```python
from build123d import *

# Parameters (mm, degrees)
BOSS_EXTRUDE1_DEPTH = 2.54
SKETCH2_R           = 3.048
SKETCH2_R_2         = 1.8669
BOSS_EXTRUDE2_DEPTH = 1.1176
FILLET1_R           = 1.143
SKETCH3_R           = 1.8669
SKETCH3_R_2         = 1.42875
BOSS_EXTRUDE3_DEPTH = 1.016
SKETCH4_R           = 1.42875
CUT_EXTRUDE1_DEPTH  = 6.474765596


with BuildPart() as part:
    # Sketch1 → Boss-Extrude1 (new body)
    with BuildSketch(Plane(origin=(0, 0, 0), x_dir=(1, 0, 0), z_dir=(0, 1, 0))):
        Polygon((3.666174209, 0), (1.833087105, 3.175), (-1.833087105, 3.175), (-3.666174209, 0), (-1.833087105, -3.175), (1.833087105, -3.175), align=None)
    extrude(amount=BOSS_EXTRUDE1_DEPTH)

    # Sketch2 → Boss-Extrude2 (add)
    with BuildSketch(Plane(origin=(0, 2.54, 0), x_dir=(1, 0, 0), z_dir=(0, 1, 0))):
        with Locations(Location((0, 0, 0), (0, 0, 270))):
            Circle(SKETCH2_R)
        with Locations(Location((0, 0, 0), (0, 0, 270))):
            Circle(SKETCH2_R_2, mode=Mode.SUBTRACT)
    extrude(amount=BOSS_EXTRUDE2_DEPTH)

    # Fillet1
    # the kernel refuses this fillet: 1.143 mm, written as the material it takes off along each edge
    with BuildSketch(Plane(origin=(0, 3.6576, 0), x_dir=(0, 0, 1), z_dir=(-1, 0, 0))) as fillet1_piece_1_section:
        with BuildLine():
            CenterArc((3.048 - FILLET1_R, -FILLET1_R), FILLET1_R, 0, 90)
            Line((3.048 - FILLET1_R, 0), (3.048, 0))
            Line((3.048, 0), (3.048, -FILLET1_R))
        make_face()
    fillet1_piece_1 = revolve(axis=Axis((0, 3.6576, 0), (0, 1, 0)), mode=Mode.PRIVATE)
    fillet1_piece_1 = split(fillet1_piece_1, bisect_by=Plane(origin=(0, 2.54, -2.716774649), z_dir=(0, 1, 0)), keep=Keep.TOP, mode=Mode.PRIVATE)
    add(fillet1_piece_1, mode=Mode.SUBTRACT)

    # Sketch3 → Boss-Extrude3 (add)
    with BuildSketch(Plane(origin=(0, 2.54, 0), x_dir=(1, 0, 0), z_dir=(0, 1, 0))):
        with Locations(Location((0, 0, 0), (0, 0, 270))):
            Circle(SKETCH3_R)
        with Locations(Location((0, 0, 0), (0, 0, 270))):
            Circle(SKETCH3_R_2, mode=Mode.SUBTRACT)
    extrude(amount=BOSS_EXTRUDE3_DEPTH)

    # Sketch4 → Cut-Extrude1 (cut, through all)
    with BuildSketch(Plane(origin=(0, 2.54, 0), x_dir=(1, 0, 0), z_dir=(0, 1, 0))):
        with Locations(Location((0, 0, 0), (0, 0, 270))):
            Circle(SKETCH4_R)
    extrude(amount=-CUT_EXTRUDE1_DEPTH, mode=Mode.SUBTRACT)


solid = part.part
```
Read the model definition and answer for the solid it produces. Units are mm, in the model's axes. Give positions to 0.01 mm unless a question says otherwise; leave off trailing zeros. Loops run counter-clockwise (first coordinate to the right, second up) from the corner with the lowest first, then second, coordinate; pieces in that order, holes last.
Item 1: Find the intervals of material crossed by line 1 along X through (y, z) = (2.2, 0.5); line 2 along Z through (x, y) = (0.75, 0.5) (3 decimals); line 3 along Y through (x, z) = (-1.5, 0), in increasing order.
Item 2: The part is cut by section C-C (x = 3.25). Write down the section's boundary in (y, z), and give its area (3 significant figures).
Item 3: The part is cut by section A-A (x = 0). Write down the section's boundary in (y, z) (3 decimals).
Item 4: Each of these flat-tipped pins is pushed along its axis until it touches: pin 1 Ø3.5 at (x, z) = (0, 0) entering from -Y; pin 2 Ø3.5 at (x, z) = (0, 0) entering from +Y; pin 3 Ø1.7 at (x, z) = (0, 0) entering from -Y. Where does it stop, or does it pass through?
Item 5: The part is cut by section B-B (y = 2.25). Write down the section's boundary in (x, z) (1 decimal), and give its area (3 significant figures).
Item 6: The part is cut by section D-D (y = 3.45). Write down the section's boundary in (x, z), and give its area (3 significant figures).
Taken from the geometry:
1. line 1: x = -3.38 to -1.34, 1.34 to 3.38
1. line 2: z = -3.175 to -1.216, 1.216 to 3.175
1. line 3: y = 0 to 3.56
2. outline: (0, -0.72) - (2.54, -0.72) - (2.54, 0.72) - (0, 0.72) - close
2. area: 3.66 mm2
3. outline: (0, -3.175) - (2.54, -3.175) - (2.54, -3.048) arc R1.143 ccw to (3.658, -1.905) - (3.658, -1.867) - (3.556, -1.867) - (3.556, -1.429) - (0, -1.429) - close; (0, 1.429) - (3.556, 1.429) - (3.556, 1.867) - (3.658, 1.867) - (3.658, 1.905) arc R1.143 ccw to (2.54, 3.048) - (2.54, 3.175) - (0, 3.175) - close
4. pin 1: stops at y = 0
4. pin 2: stops at y = 3.56
4. pin 3: passes through
5. outline: (-3.7, 0) - (-1.8, -3.2) - (1.8, -3.2) - (3.7, 0) - (1.8, 3.2) - (-1.8, 3.2) - close; hole circle Ø2.9 at (0, 0)
5. area: 28.5 mm2
6. outline: circle Ø5.12 at (0, 0); hole circle Ø2.86 at (0, 0)
6. area: 14.2 mm2
